For this review, take the finished solid that the model builds, in its own axes (mm). Face numbers are marked on the shaded views. A direction names the side the tool comes from. Give positions to 0.01 mm unless a question says otherwise; leave off trailing zeros. Loops run counter-clockwise (first coordinate to the right, second up) from the corner with the lowest first, then second, coordinate; pieces in that order, holes last. Notation, with made-up numbers: (45.25, 42) - (75.25, 42) arc R25 ccw to (75.25, 58) - close; hole circle Ø11 at (76, 39). An arc over 180 degrees is marked (long way). Use CSV: the item, a comma, the result in double quotes. Start each with the question number.
1. Take a section at B-B on z = 3. Give the boundary of the cut face in (x, y), plus the area to 3 significant figures.
2. Take a section at C-C on y = -12. Give the boundary of the cut face in (x, z).
3. Take a section at D-D on x = -55.5. Give the boundary of the cut face in (y, z).
4. Wall thickness on line 1 (X direction, y = 2.5, z = -19); line 2 (Z direction, x = 11, y = -22.5); line 3 (Y direction, x = -111, z = -8): over which ranges is each line inside the solid? List them lowest first.
5. For pin 1 (5 mm diameter, centred on x = -108.5, z = -11.5, fed in from +Y); pin 2 (13 mm diameter, centred on x = 2.5, z = -25.5, fed in from -Y) (3 decimals); pin 3 (4 mm diameter, centred on x = 16.5, z = -12.5, fed in from -Y); pin 4 (5 mm diameter, centred on x = -46, y = 8.5, fed in from -Z), all flat-tipped, find the tip position at first contact; note any pin that passes through.
6. For the marked faces 1, 2 and 3, list the 3-axis set-ups (+Z, -Z, +X, -X, +Y, -Y) from which the entire face can be reached by the end or side of a thin tool; tool diameter is ignored.
```python
from build123d import *

# Parameters (mm, degrees)
F0_R      = 38.1
F1_DEPTH  = 7.874
F2_R      = 27.4701
F3_DEPTH  = 16.51
F4_R      = 4.7244
F5_DEPTH  = 110.8964
F6_DEPTH  = 80.4672
F7_R      = 2.2352
F8_DEPTH  = 58.293
F9_W      = 16.002
F9_H      = 6.35
F10_DEPTH = 19.177
F11_R     = 8.00099
F13_D     = 6.35


# Not quite as in the source:
# - a fillet or chamfer is up to 0.001 mm smaller than in the source, because OpenCascade refuses the exact size


with BuildPart() as f1:
    # F0 (on Top) → F1 (new body)
    with BuildSketch(Plane.XY):
        Circle(F0_R)
    extrude(amount=F1_DEPTH)

    # F2 (on Top) → F3 (join)
    with BuildSketch(Plane.XY):
        Circle(F2_R)
    extrude(amount=-F3_DEPTH)

    # F4 (on Right) → F5 (join)
    with BuildSketch(Plane.YZ):
        with Locations((0, -8.4328)):
            Circle(F4_R)
    extrude(amount=F5_DEPTH)

    # F4 (on Right) → F6 (join)
    with BuildSketch(Plane.YZ):
        with Locations((0, -8.4328)):
            Circle(F4_R)
    extrude(amount=-F6_DEPTH)

    # F7 (on face) → F8 (join)
    with BuildSketch(Plane(origin=(-80.4672, 0, 0), x_dir=(0, -1, 0), z_dir=(-1, 0, 0))):
        with Locations((0, -8.4328)):
            Circle(F7_R)
    extrude(amount=F8_DEPTH)

    # F9 (on face) → F10 (join)
    with BuildSketch(Plane(origin=(0, 0, -16.51), x_dir=(1, 0, 0), z_dir=(0, 0, -1))):
        Rectangle(F9_W, F9_H)
    extrude(amount=F10_DEPTH)

    # F11 (radius 8.001 in the source; OpenCascade refuses exactly that, so slightly less here)
    f11_edges = [f1.edges().sort_by_distance(p)[0] for p in [
        (8.001, 0, -35.687),
        (-8.001, 0, -35.687),
    ]]
    fillet(f11_edges, radius=F11_R)

    # F13 (through all)
    with Locations(Plane(origin=(0, 3.175, 0), x_dir=(-1, 0, 0), z_dir=(0, 1, 0))):
        with Locations((0, -27.686)):
            Hole(F13_D / 2)


solid = f1.part
```
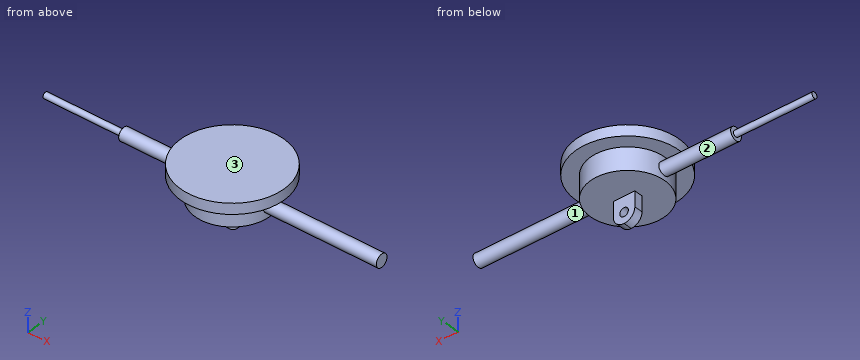
Check result:
1,outline,"circle Ø76.2 at (0, 0)"
1,area,"4,560 mm²"
2,outline,"(-36.16, 0) - (-24.71, 0) - (-24.71, -16.51) - (24.71, -16.51) - (24.71, 0) - (36.16, 0) - (36.16, 7.87) - (-36.16, 7.87) - close"
3,outline,"circle Ø9.45 at (0, -8.43)"
4,line 1,"x = -8 to 8"
4,line 2,"z = -16.51 to 7.87"
4,line 3,"y = -2.19 to 2.19"
5,pin 1,"stops at y = 2.16"
5,pin 2,"stops at y = -3.175"
5,pin 3,"stops at y = -23.33"
5,pin 4,"passes through"
6,face 1,"+X"
6,face 2,"-X"
6,face 3,"+Z, +X, -X, +Y, -Y"
